Drawing for the job (mm, zero at the part's lowest x, y, z). A direction names the side the tool comes from. Round coordinates to 2 decimals unless told otherwise and drop trailing zeros. Order: outer loops, then holes, each group sorted by start corner. A loop starts at its lowest first (then second) coordinate and runs counter-clockwise, first axis right, second up. Notation, with made-up numbers: M 85.5,51.5 L 94.5,51.5 A20 cw 94.5,81.5 Z; hole C -8.5,-30.5 d9. An arc over 180 degrees is marked long. One line per item, written item: value. Start each with the question number.
Item 1: Band-saw the part on A-A, the plane y = 17.25. Write the cut outline in (x, z), then the cut area to 3 significant figures.
Item 2: Pin check, flat tips, straight feed: pin 1 (4 mm diameter, centred on y = 15.5, z = 9, fed in from +X); pin 2 (2.5 mm diameter, centred on x = 6.64, z = 5.75, fed in from -Y); pin 3 (4 mm diameter, centred on x = 11, y = 23.5, fed in from +Z); pin 4 (1.5 mm diameter, centred on y = 11, z = 2.5, fed in from -X). Stop position of each tip, or through.
Item 3: Tool access for the marked faces 5 and 6: list every direction of +Z, -Z, +X, -X, +Y, -Y with a clear straight run to the whole face (end or side of a thin tool).
Item 4: Probe L1, parallel to X at y = 19, z = 5.75; L2, parallel to Z at x = 6.75, y = 11.75; L3, parallel to Z at x = 6.5, y = 2.5 (1 decimal). List the from-to ranges inside material, lowest first.
Item 5: Two-plate mould, pull along X, no slides. Class the marked faces 1, 2, 3 and 4: +X half, -X half, draft (parallel to the pull), parting line (faces both ways), or undercut.
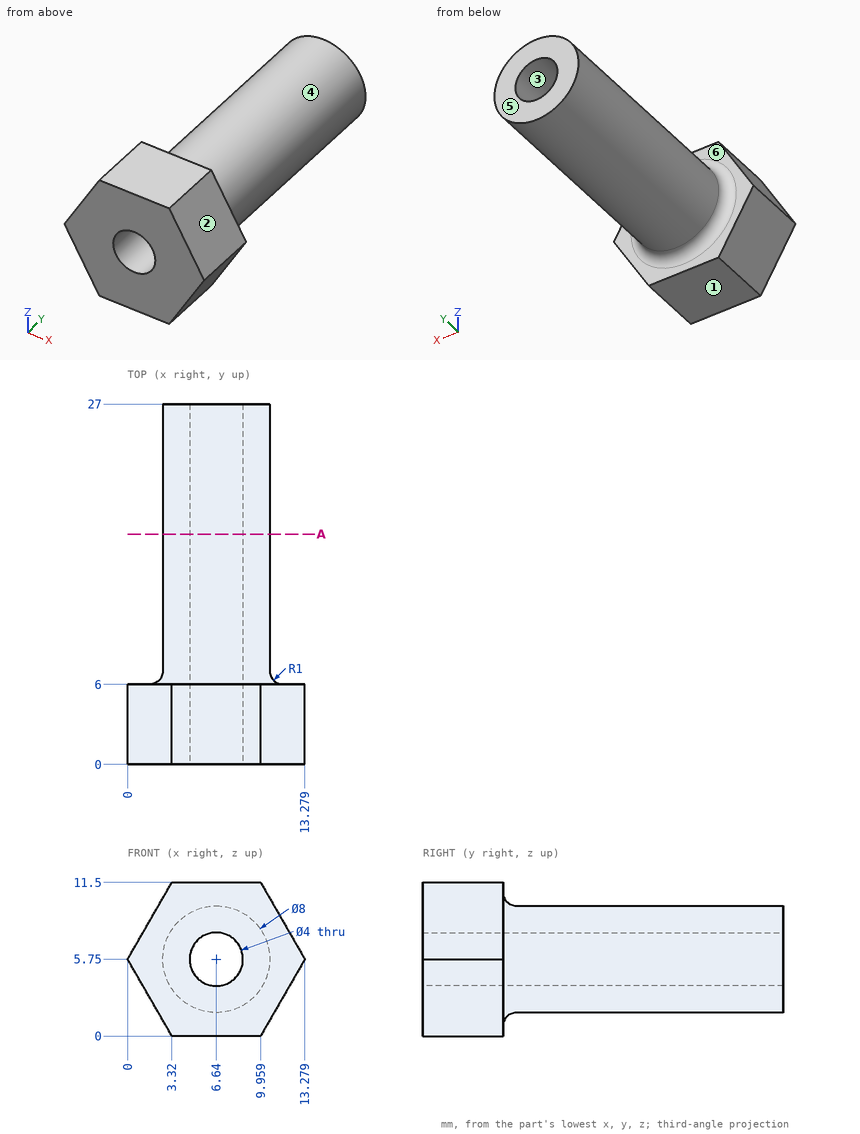
Output:
1. outline: C 6.64,5.75 d8; hole C 6.64,5.75 d4
1. area: 37.7 mm²
2. pin 1: stops at x = 10.44
2. pin 2: passes through
2. pin 3: stops at z = 8.98
2. pin 4: stops at x = 3.52
3. face 5: +Z, -Z, +X, -X, +Y
3. face 6: +Y
4. L1: x = 2.64 to 4.64, 8.64 to 10.64
4. L2: z = 1.75 to 3.75, 7.75 to 9.75
4. L3: z = 0 to 3.8, 7.7 to 11.5
5. face 1: draft
5. face 2: +X half
5. face 3: undercut
5. face 4: parting line
